Part model, mm, in its own coordinate system. A direction names the side the tool comes from. Round coordinates to 2 decimals unless told otherwise and drop trailing zeros. Write each loop counter-clockwise with the first axis right and the second up, starting at its lowest first coordinate (ties: lowest second). Pieces come first, ordered by that corner, then holes. Notation, with made-up numbers: (29.25, 6) -> (36.25, 6) arc R24 cw to (36.25, 20) -> close; hole circle Ø3 at (33, -38). An arc over 180 degrees is marked (long way). Return JSON: item names as keys, results as strings. Group by question number.
(1) Mould opens along X. For faces 1 (the flat face through (10, 0, 0)), 2 (the cylindrical face through (26.448, -2.589, 5.3)), 3 (the flat face through (29.35, 0, 5)) say: +X half, -X half, draft (parallel to the pull), parting line (faces both ways), or undercut.
(2) Drill centre lines: L1, parallel to X at y = -15, z = 1.5; L2, parallel to X at y = 13.5, z = 0.5; L3, parallel to X at y = -1.5, z = 7.75. Where is each one in solid material? Low to high. Write a range as from..to.
(3) Tool access for faces 4 (the cylindrical face through (-9.2, 19.13, 1.01)), 5 (the cylindrical face through (-9.23, -19.1, 1.01)), 6 (the cylindrical face through (26.403, 13.342, 5.3)), 7 (the cylindrical face through (28.78, 19.1, 5.45)), 8 (the flat face through (-9.8, 0, 1)): list every direction of +Z, -Z, +X, -X, +Y, -Y with a clear straight run to the whole face (end or side of a thin tool).
(4) Saw through at B-B (y = -9.5). List the corners of the cut face in (x, z), plus the area to 3 significant figures.
(5) Saw through at A-A (x = -20). List the corners of the cut face in (y, z), plus the area to 3 significant figures.
(6) Drop flat-ended pins along their axis: pin 1 Ø1.4 at (x, y) = (25.81, -2.1) entering from +Z; pin 2 Ø11 at (x, y) = (-20, 9) entering from -Z. Give the stop position or say it passes through.
Autodesk Inventor part; units mm, degrees
ref_plane "YZ Plane" through (0, 0, 0) normal (1, 0, 0) x (0, 1, 0)
ref_plane "XZ Plane" through (0, 0, 0) normal (0, 1, 0) x (-1, 0, 0)
ref_plane "XY Plane" through (0, 0, 0) normal (0, 0, 1) x (1, 0, 0)
sketch "Sketch1" plane through (0, 0, 0) normal (0, 0, 1) x (1, 0, 0)
  line L0 (-29.35, -19.7) -> (29.35, -19.7)
  line L1 (29.35, -19.7) -> (29.35, 19.7)
  line L2 (29.35, 19.7) -> (-29.35, 19.7)
  line L3 (-29.35, 19.7) -> (-29.35, -19.7)
  line L4 (-29.35, -19.7) -> (29.35, 19.7) construction
  line L5 (29.35, -19.7) -> (-29.35, 19.7) construction
  point P0 (0, 0)
  dimension "d0" = 39.4
  dimension "d1" = 58.7
extrude "Extrusion1" add sketch "Sketch1" along normal blind 10.75
sketch "Sketch2" plane through (0, 0, 0) normal (0, 0, -1) x (-1, 0, 0)
  circle A0 centre (7.6129, -2.1018) radius 1.5 construction
  circle A1 centre (-25.8129, -2.1018) radius 1.5 construction
  circle A2 centre (-25.8129, 12.8018) radius 1.5 construction
  circle A3 centre (7.6129, 12.8018) radius 1.5 construction
  circle A4 centre (7.6129, -2.1018) radius 0.8
  circle A5 centre (-25.8129, -2.1018) radius 0.8
  circle A6 centre (-25.8129, 12.8018) radius 0.8
  circle A7 centre (7.6129, 12.8018) radius 0.8
  point P0 (0, 0)
  dimension "d4" = 1.6
  dimension "d5" = 1.6
  dimension "d6" = 1.6
  dimension "d7" = 1.6
extrude "Extrusion2" cut sketch "Sketch2" against normal through all
sketch "Sketch5" plane through (0, 0, 0) normal (0, 0, -1) x (-1, 0, 0)
  line L0 (-29.35, 19.7) -> (29.35, 19.7)
  line L1 (29.35, -19.7) -> (9.8, -19.7)
  line L2 (9.8, -19.7) -> (9.8, 19.7)
  line L3 (9.8, 19.7) -> (29.35, 19.7)
  line L4 (29.35, 19.7) -> (29.35, -19.7)
  point P0 (0, 0)
  dimension "d10" = 19.55
extrude "Extrusion3" cut sketch "Sketch5" against normal blind 2
fillet "Fillet1" radius 2 4 edges at (-29.35, -19.7, 6.375) (-29.35, 19.7, 6.375) (29.35, 19.7, 5.375) (29.35, -19.7, 5.375)
fillet "Fillet2" radius 2 2 edges at (-9.8, 19.7, 1) (-9.8, -19.7, 1)
equation "\"d5\" = d4"
equation "\"d6\" = d4"
equation "\"d7\" = d4"
properties part number "ThermalConductivityBlock"
Computed values:
{
 "1": {"face 1": "draft", "face 2": "undercut", "face 3": "+X half"},
 "2": {"L1": "-9.8..29.35", "L2": "-9.8..-8, -7.22..25.42, 26.2..29.35", "L3": "-29.35..-8.14, -7.09..25.29, 26.34..29.35"},
 "3": {"face 4": "-Z, -X, +Y", "face 5": "-Z, -X, -Y", "face 6": "+Z, -Z", "face 7": "+Z, -Z, +X, +Y", "face 8": "-Z, -X, +Y, -Y"},
 "4": {"outline": "(-29.35, 2) -> (-9.8, 2) -> (-9.8, 0) -> (29.35, 0) -> (29.35, 10.75) -> (-29.35, 10.75) -> close", "area": "592 mm2"},
 "5": {"outline": "(-19.7, 2) -> (19.7, 2) -> (19.7, 10.75) -> (-19.7, 10.75) -> close", "area": "345 mm2"},
 "6": {"pin 1": "through", "pin 2": "z = 2"}
}
